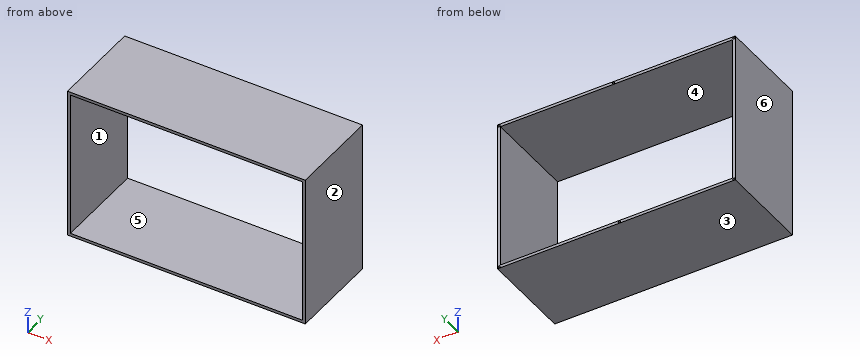
from build123d import *

# Parameters (mm, degrees)
SKETCH5_W                = 246
SKETCH5_H                = 158
SKETCH5_W_2              = 240
SKETCH5_H_2              = 152
BOSS_EXTRUDE1_DEPTH      = 95
M2_CLEARANCE_HOLE1_D     = 2.4
M2_CLEARANCE_HOLE1_DEPTH = 3
M2_CLEARANCE_HOLE1_TIP   = 0.721032743


with BuildPart() as part:
    # Sketch5 → Boss-Extrude1 (new body)
    with BuildSketch(Plane(origin=(0, 0, 0), x_dir=(1, 0, 0), z_dir=(0, 1, 0))):
        Rectangle(SKETCH5_W, SKETCH5_H)
        Rectangle(SKETCH5_W_2, SKETCH5_H_2, mode=Mode.SUBTRACT)
    extrude(amount=BOSS_EXTRUDE1_DEPTH)

    # M2 Clearance Hole1
    with Locations(Plane(origin=(-121.5, 95, -77.5), x_dir=(0, 0, 1), z_dir=(0, 1, 0))):
        with Locations((0, 0), (155, 0), (155, 243), (0, 243), (0, 118.5), (155, 124.5)):
            Hole(M2_CLEARANCE_HOLE1_D / 2, depth=M2_CLEARANCE_HOLE1_DEPTH)
            with Locations((0, 0, -(M2_CLEARANCE_HOLE1_DEPTH + M2_CLEARANCE_HOLE1_TIP / 2))):  # 118° drill point
                Cone(0, M2_CLEARANCE_HOLE1_D / 2, M2_CLEARANCE_HOLE1_TIP, mode=Mode.SUBTRACT)


solid = part.part
Could you check a few things on this model? Use its own coordinates, in mm. Face numbers are marked on the shaded views. A direction names the side the tool comes from. Round coordinates to 2 decimals unless told otherwise and drop trailing zeros. Loops run counter-clockwise (first coordinate to the right, second up) from the corner with the lowest first, then second, coordinate; pieces in that order, holes last. Notation, with made-up numbers: (30, -27) -> (71, -27) arc R30 cw to (71, 11) -> close; hole circle Ø11 at (74, -20.5). An arc over 180 degrees is marked (long way). Use CSV: the item, a comma, the result in double quotes.
(1) If I drill on probe 1 along X at (y, z) = (94.4, 77.5); probe 2 along Z at (x, y) = (-3, 92); probe 3 along Z at (x, y) = (109, 22), over which ranges is the centre line in solid material (lowest first)? Write a range as [from, to].
Return value:
probe 1,"x = [-123, -122.7], [-120.3, 1.8], [4.2, 120.3], [122.7, 123]"
probe 2,"z = [-79, -78.7], [-76.3, -76], [76, 79]"
probe 3,"z = [-79, -76], [76, 79]"
(2) If we mould it in two halves opening along Z, with no side actions, what happens to the marked faces 1, 2, 3 and 4? For each: +Z half, -Z half, draft (parallel to the pull), parting line (faces both ways), or undercut.
Return value:
face 1,"undercut"
face 2,"draft"
face 3,"-Z half"
face 4,"undercut"
(3) Suppose I cut it at B-B on x = 45. Write out the boundary of the cut face in (y, z).
Return value:
outline,"(0, -79) -> (95, -79) -> (95, -76) -> (0, -76) -> close; (0, 76) -> (95, 76) -> (95, 79) -> (0, 79) -> close"
(4) Suppose I cut it at C-C on y = 20. Write out the boundary of the cut face in (x, z).
Return value:
outline,"(-123, -79) -> (123, -79) -> (123, 79) -> (-123, 79) -> close; hole (-120, -76) -> (120, -76) -> (120, 76) -> (-120, 76) -> close"
(5) Will this pin go through, and if not, where does the flat tip stop? pin 1 Ø1.4 at (x, z) = (121.5, 77.5) entering from +Y.
Return value:
pin 1,"stops at y = 91.7"
(6) Suppose I cut it at A-A on z = 66. Write out the boundary of the cut face in (x, y), plus the area to 3 significant figures.
Return value:
outline,"(-123, 0) -> (-120, 0) -> (-120, 95) -> (-123, 95) -> close; (120, 0) -> (123, 0) -> (123, 95) -> (120, 95) -> close"
area,"570 mm²"
(7) For the marked faces 5 and 6, which set-ups out of +Z, -Z, +X, -X, +Y, -Y let a thin tool reach every point of the face, with its end or its side?
Return value:
face 5,"+Y, -Y"
face 6,"+Z, -Z, -X, +Y, -Y"
